from build123d import *

# Parameters (mm, degrees)
SKETCH1_R           = 2
BOSS_EXTRUDE3_DEPTH = 5
CHAMFER2_SIZE       = 0.5
CUT_EXTRUDE2_DEPTH  = 2


with BuildPart() as part:
    # Sketch1 → Boss-Extrude3 (new body)
    with BuildSketch(Plane(origin=(0, 0, 0), x_dir=(1, 0, 0), z_dir=(0, 1, 0))):
        Circle(SKETCH1_R)
    extrude(amount=-BOSS_EXTRUDE3_DEPTH)

    # Sketch3 → Revolve2 (revolve)
    with BuildSketch(Plane.XY):
        with BuildLine():
            Line((-3.5, 0), (-3.5, 0.3))
            ThreePointArc((-3.5, 0.3), (-1.988393808, 1.6859585), (0, 2.188078318))
            Line((0, 2.188078318), (0, 0))
            Line((0, 0), (-3.5, 0))
        make_face()
    revolve(axis=Axis((0, -2, 0), (0, 1, 0)))

    # Chamfer2
    chamfer2_edges = [part.edges().sort_by_distance(p)[0] for p in [
        (-2, -5, 0),
    ]]
    chamfer(chamfer2_edges, length=CHAMFER2_SIZE)

    # Sketch4 → Cut-Extrude2 (cut)
    with BuildSketch(Plane(origin=(0, 2.188078318, 0), x_dir=(1, 0, 0), z_dir=(0, 1, 0))):
        Polygon((0, 1.732050808), (-1.5, 0.866025404), (-1.5, -0.866025404), (0, -1.732050808), (1.5, -0.866025404), (1.5, 0.866025404), align=None)
    extrude(amount=-CUT_EXTRUDE2_DEPTH, mode=Mode.SUBTRACT)


solid = part.part
The model under review builds one solid part; all positions refer to its coordinate system, in mm. A direction names the side the tool comes from. Give positions to 0.01 mm unless a question says otherwise; leave off trailing zeros. Order: outer loops, then holes, each group sorted by start corner. A loop starts at its lowest first (then second) coordinate and runs counter-clockwise, first axis right, second up. Notation, with made-up numbers: (-34.5, 51) -> (-9.5, 51) arc R35 ccw to (-9.5, 88) -> close; hole circle Ø8 at (42.25, 6). An arc over 180 degrees is marked (long way). Write item = value, one per line. Start each with the question number.
(1) Take a section at C-C (x = 2.5). Write out the cut boundary in (y, z).
(2) Take a section at B-B (y = -1.5). Write out the cut boundary in (x, z).
(3) For L1, parallel to Y at x = -0.5, z = 1.25; L2, parallel to Z at x = -1, y = -0.75, list the stretches that pass through material, from the lowest coordinate up. Write a range as from..to.
(4) Tool access review of faces 4 (the cylindrical face through (-3.34, 0.15, 1.05)), 5 (the flat face through (2, 0, -2)), 6 (the flat face through (0, 0.188, 0)): name each direction out of +Z, -Z, +X, -X, +Y, -Y from which nothing blocks a thin tool from reaching the whole face with its end or side.
(5) For pin 1 Ø1.5 at (y, z) = (-2, -0.5) entering from -X; pin 2 Ø4 at (y, z) = (-3, 0.5) entering from +X; pin 3 Ø3 at (y, z) = (-1, -1.5) entering from -X, all flat-tipped, find the tip position at first contact; note any pin that passes through.
(6) Draft analysis for pull direction Z (two halves, no side actions). For faces 1 (the cylindrical face through (0, -2, 2)), 2 (the flat face through (-1.5, 1, 0)), 3 (the flat face through (0, -5, 0)), state which applies: +Z half, -Z half, draft (parallel to the pull), parting line (faces both ways), or undercut.
(7) Take a section at A-A (z = 0). Write out the cut boundary in (x, y).
Returned:
q1.outline = (0, -2.45) -> (0.3, -2.45) arc R3.36 ccw to (0.3, 2.45) -> (0, 2.45) -> close
q2.outline = circle Ø4 at (0, 0)
q3.L1 = -5..0.19
q3.L2 = -1.73..1.73
q4.face_4 = +Y, -Y
q4.face_5 = -Y
q4.face_6 = +Y
q5.pin_1 = -2
q5.pin_2 = 2
q5.pin_3 = -3.48
q6.face_1 = parting line
q6.face_2 = undercut
q6.face_3 = draft
q7.outline = (-3.5, 0) -> (-2, 0) -> (-2, -4.5) -> (-1.5, -5) -> (1.5, -5) -> (2, -4.5) -> (2, 0) -> (3.5, 0) -> (3.5, 0.3) arc R4.19 ccw to (1.5, 1.91) -> (1.5, 0.19) -> (-1.5, 0.19) -> (-1.5, 1.91) arc R4.19 ccw to (-3.5, 0.3) -> close
